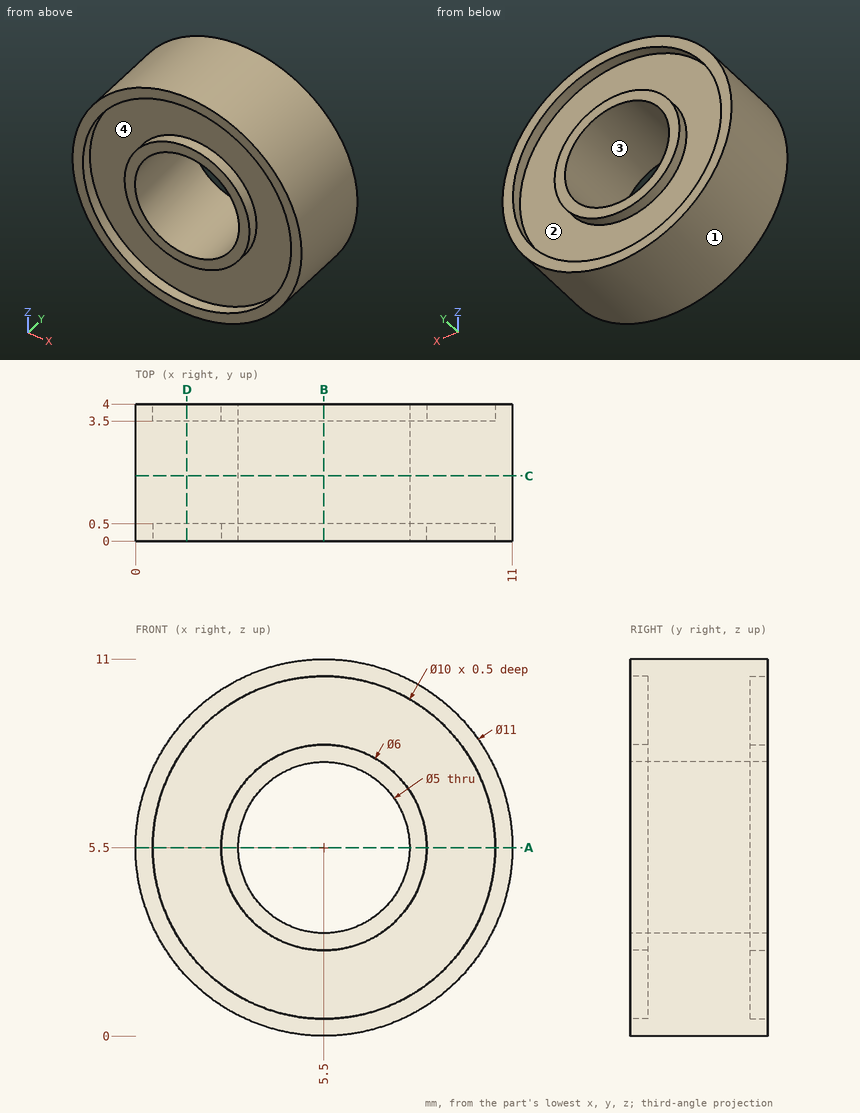
Verification items for this drawing (mm, ordinates from the low corner). A direction names the side the tool comes from. Give positions to 0.01 mm unless a question says otherwise; leave off trailing zeros. Write each loop counter-clockwise with the first axis right and the second up, starting at its lowest first coordinate (ties: lowest second). Pieces come first, ordered by that corner, then holes. Notation, with made-up numbers: (8.25, 36) -> (13.25, 36) arc R31 cw to (13.25, 70) -> close; hole circle Ø3 at (40, 62). An arc over 180 degrees is marked (long way). Write item = value, one per line.
Item 1: Scan lines: probe 1 along Z at (x, y) = (5.5, 3.65); probe 2 along Z at (x, y) = (4.75, 0.35); probe 3 along Z at (x, y) = (5.5, 0.8). Record each from-to range of solid material in increasing order. Write a range as from..to.
Output:
probe_1 = 0..0.5, 2.5..3, 8..8.5, 10.5..11
probe_2 = 0.05..0.56, 2.6..3.12, 7.88..8.4, 10.44..10.95
probe_3 = 0..3, 8..11
Item 2: Release check for a two-part mould opening along Z. For the marked faces 1 and 2 record: +Z half, -Z half, draft (parallel to the pull), parting line (faces both ways), or undercut.
Output:
face_1 = parting line
face_2 = undercut
Item 3: Sectioned sample at C-C on y = 1.9. Record the boundary of the cut face in (x, z).
Output:
outline = circle Ø11 at (5.5, 5.5); hole circle Ø5 at (5.5, 5.5)
Item 4: Sectioned sample at D-D on x = 1.5. Record the boundary of the cut face in (y, z).
Output:
outline = (0, 1.73) -> (4, 1.73) -> (4, 2.5) -> (3.5, 2.5) -> (3.5, 8.5) -> (4, 8.5) -> (4, 9.27) -> (0, 9.27) -> (0, 8.5) -> (0.5, 8.5) -> (0.5, 2.5) -> (0, 2.5) -> close
Item 5: Sectioned sample at B-B on x = 5.5. Record the boundary of the cut face in (y, z), and give its area (3 significant figures).
Output:
outline = (0, 0) -> (4, 0) -> (4, 0.5) -> (3.5, 0.5) -> (3.5, 2.5) -> (4, 2.5) -> (4, 3) -> (0, 3) -> (0, 2.5) -> (0.5, 2.5) -> (0.5, 0.5) -> (0, 0.5) -> close; (0, 8) -> (4, 8) -> (4, 8.5) -> (3.5, 8.5) -> (3.5, 10.5) -> (4, 10.5) -> (4, 11) -> (0, 11) -> (0, 10.5) -> (0.5, 10.5) -> (0.5, 8.5) -> (0, 8.5) -> close
area = 20.0 mm^2
Item 6: Sectioned sample at A-A on z = 5.5. Record the boundary of the cut face in (x, y).
Output:
outline = (0, 0) -> (0.5, 0) -> (0.5, 0.5) -> (2.5, 0.5) -> (2.5, 0) -> (3, 0) -> (3, 4) -> (2.5, 4) -> (2.5, 3.5) -> (0.5, 3.5) -> (0.5, 4) -> (0, 4) -> close; (8, 0) -> (8.5, 0) -> (8.5, 0.5) -> (10.5, 0.5) -> (10.5, 0) -> (11, 0) -> (11, 4) -> (10.5, 4) -> (10.5, 3.5) -> (8.5, 3.5) -> (8.5, 4) -> (8, 4) -> close
Item 7: Tool access check on the marked faces 3 and 4. Record the directions out of +Z, -Z, +X, -X, +Y, -Y that give a thin tool (end or side, any length) a straight path to the whole face; none if there is none.
Output:
face_3 = +Y, -Y
face_4 = -Y
Item 8: Gauge pin test, flat ends, axial feed: pin 1 (2 mm diameter, centred on x = 3, y = 2.5, fed in from -Z); pin 2 (1.5 mm diameter, centred on y = 2, z = 7, fed in from -X). Record the tip position at first contact, or that the pin passes through.
Output:
pin_1 = 0.21
pin_2 = 0.05
